The model under review builds one solid part; all positions refer to its coordinate system, in mm. Coordinates: 2 decimals unless noted, no trailing zeros. Order: outer loops, then holes, each group sorted by start corner. A loop starts at its lowest first (then second) coordinate and runs counter-clockwise, first axis right, second up.
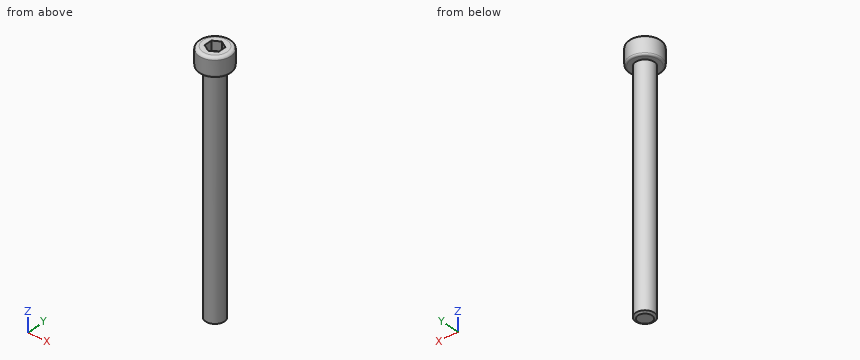
```python
from build123d import *

# Parameters (mm, degrees)
CHAMFER_1_SIZE      = 0.3
CHAMFER_1_SIZE2     = 0.519615242
FILLET_1_R          = 0.4
FILLET_2_SIZE       = 0.5
FILLET_2_SIZE_2     = 0.8
CUT_EXTRUDE_1_DEPTH = 2


with BuildPart() as part:
    # 草图2 → 旋转1 (revolve)
    with BuildSketch(Plane(origin=(0, 0, 0), x_dir=(0, 0, -1), z_dir=(1, 0, 0)), mode=Mode.PRIVATE) as revolve_1_sk:
        Polygon((-27, 0), (-27, 3.4), (-23, 3.4), (-23, 2), (27, 2), (27, 0), align=None)
    revolve(revolve_1_sk.sketch.rotate(Axis((0, 0, -27), (0, 0, 1)), 90), axis=Axis((0, 0, -27), (0, 0, 1)))

    # 倒角1
    chamfer_1_edges = [part.edges().sort_by_distance(p)[0] for p in [
        (2, 0, -27),
    ]]
    chamfer_1_side = [part.faces().sort_by_distance(p)[0] for p in [
        (2, 0, -2),
    ]]
    chamfer(chamfer_1_edges, length=CHAMFER_1_SIZE, length2=CHAMFER_1_SIZE2, reference=chamfer_1_side[0])

    # 圆角1
    fillet_1_edges = [part.edges().sort_by_distance(p)[0] for p in [
        (3.4, 0, 23),
    ]]
    fillet(fillet_1_edges, radius=FILLET_1_R)

    # 圆角2
    # an asymmetric fillet: 0.8, 0.5 mm, written as the material it takes off along each edge
    with BuildSketch(Plane(origin=(0, 0, 27), x_dir=(-1, 0, 0), z_dir=(0, 1, 0))) as fillet_2_piece_1:
        with BuildLine():
            Bezier((3.4, -FILLET_2_SIZE), (3.4, 0), (3.4 - FILLET_2_SIZE_2, 0), weights=[1, 0.707106781, 1])
            Line((3.4 - FILLET_2_SIZE_2, 0), (3.4, 0))
            Line((3.4, 0), (3.4, -FILLET_2_SIZE))
        make_face()
    revolve(axis=Axis((0, 0, 27), (0, 0, 1)), mode=Mode.SUBTRACT)

    # 草图3 → 切除-拉伸1 (cut)
    with BuildSketch(Plane.XY.offset(27)):
        Polygon((0, 1.732050808), (-1.5, 0.866025404), (-1.5, -0.866025404), (0, -1.732050808), (1.5, -0.866025404), (1.5, 0.866025404), align=None)
    extrude(amount=-CUT_EXTRUDE_1_DEPTH, mode=Mode.SUBTRACT)


solid = part.part
```
(1) For pin 1 Ø3 at (y, z) = (0.5, -21) entering from +X; pin 2 Ø4 at (x, z) = (0, 20) entering from +Y; pin 3 Ø1.5 at (y, z) = (-2.5, -9.5) entering from +X, all flat-tipped, find the tip position at first contact; note any pin that passes through.
A:
pin 1: stops at x = 2
pin 2: stops at y = 2
pin 3: stops at x = 0.97
(2) Wall thickness on probe 1 along Z at (x, y) = (0.5, 1); probe 2 along X at (y, z) = (1, 17.5); probe 3 along Z at (x, y) = (0.5, 2.5): over which ranges is each line inside the solid? List them lowest first.
A:
probe 1: z = -27 to 25
probe 2: x = -1.73 to 1.73
probe 3: z = 23 to 27
(3) We need section A-A, the plane z = -12. Write out the cut boundary in (x, y), and give its area (3 significant figures).
A:
outline: circle Ø4 at (0, 0)
area: 12.6 mm2
